Geometry check sheet. Reference: the model listing, model coordinates, mm. A direction names the side the tool comes from. Give positions to 0.01 mm unless a question says otherwise; leave off trailing zeros. Write each loop counter-clockwise with the first axis right and the second up, starting at its lowest first coordinate (ties: lowest second). Pieces come first, ordered by that corner, then holes.
(1) Mould release check, pull along X, two halves, no side actions. Record for faces 3 (the cylindrical face through (-0.586, 3.815, -12.522)), 4 (the cylindrical face through (-22.8, 0.2, -12.5)), 5 (the flat face through (-23, -1, -25.4)): +X half, -X half, draft (parallel to the pull), parting line (faces both ways), or undercut.
(2) Thickness scan on line 1 along X through (y, z) = (-11.5, 23); line 2 along X through (y, z) = (0.5, -2); line 3 along Y through (x, z) = (-12.7, 0.85). Record the ranges inside material, lowest first.
(3) Depth check by flat-ended pin: P1, Ø4, axis at y = -2, z = -11.5, coming from the +X side; P2, Ø12, axis at y = 32.5, z = 28, coming from the -X side; P3, Ø5, axis at x = 21.5, y = -3.5, coming from the -Z side; P4, Ø6, axis at y = -20, z = 2, coming from the -X side. Enter the tip coordinate at first touch or a pass-through.
(4) Tool access check on faces 1 (the conical face through (-28.38, 0.69, 8.13)), 2 (the flat face through (-2.7, -1.5, 0)). Record the directions out of +Z, -Z, +X, -X, +Y, -Y that give a thin tool (end or side, any length) a straight path to the whole face; none if there is none.
(5) Cross-section at A-A (y = 0). Record the boundary of the cut face in (x, z), and give its area (3 significant figures).
(6) Cross-section at D-D (z = 18). Record the boundary of the cut face in (x, y).
(7) Cross-section at B-B (z = 8). Record the boundary of the cut face in (x, y), and give its area (3 significant figures).
```python
from build123d import *

# Parameters (mm, degrees)
F2_R     = 10.16
F3_DEPTH = 50.8
F4_R     = 10.16
F5_DEPTH = 25.4
F6_DEPTH = 25.4


with BuildPart() as f1:
    # F0 (on Front) → F1 (revolve)
    with BuildSketch(Plane.XZ):
        Polygon((0, 0), (35.9210230905, 35.921025878), (33.2881103987, 38.4245585941), (-2.765778685, 2.3706667125), (-12.7, 2.3706667125), (-12.7, -25.4), (0, -25.4), align=None)
    revolve(axis=Axis((-12.7, 0, -11.5146666437), (0, 0, 1)))

    # F2 (on Top) → F3 (cut)
    with BuildSketch(Plane.XY):
        with Locations((-12.6435561106, 0)):
            Circle(F2_R)
    extrude(amount=-F3_DEPTH, mode=Mode.SUBTRACT)

    # F4 (on Top) → F5 (cut)
    with BuildSketch(Plane.XY):
        with Locations((-12.4460002407, 0)):
            Circle(F4_R)
    extrude(amount=-F5_DEPTH, mode=Mode.SUBTRACT)

    # F6 (cut): a face of the model
    f6_faces = [f1.faces().sort_by_distance(p)[0] for p in [
        (-12.7, 0, 2.3706667125),
    ]]
    extrude(f6_faces, amount=-F6_DEPTH, mode=Mode.SUBTRACT)


solid = f1.part
```
Reply:
1. face 3: parting line
1. face 4: undercut
1. face 5: draft
2. line 1: x = -46.5 to -41.02, 15.62 to 21.1
2. line 2: x = -25.39 to -22.79, -2.3 to -0.01
2. line 3: y = -13.55 to -9.93, 9.93 to 13.55
3. P1: stops at x = 0
3. P2: stops at x = -47.87
3. P3: stops at z = 19.18
3. P4: passes through
4. face 1: +Z
4. face 2: -Z
5. outline: (-61.32, 35.92) - (-25.4, 0) - (-25.4, -25.4) - (-22.8, -25.4) - (-22.8, 0) - (-22.63, 0) - (-22.63, 2.37) - (-58.69, 38.42) - close; (-2.77, 0) - (-2.29, 0) - (-2.29, -25.4) - (0, -25.4) - (0, 0) - (35.92, 35.92) - (33.29, 38.42) - (-2.77, 2.37) - close
5. area: 500 mm2
6. outline: circle Ø61.4 at (-12.7, 0); hole circle Ø51.13 at (-12.7, 0)
7. outline: circle Ø41.4 at (-12.7, 0); hole circle Ø31.13 at (-12.7, 0)
7. area: 585 mm2
